from build123d import *

# Parameters (mm, degrees)
SKETCH1_W           = 42
SKETCH1_H           = 47
BOSS_EXTRUDE1_DEPTH = 5
SKETCH2_R           = 1.5
SKETCH2_R_2         = 12.5
CUT_EXTRUDE1_DEPTH  = 32.910029771
SKETCH4_W           = 42
SKETCH4_H           = 45
BOSS_EXTRUDE2_DEPTH = 5
BOSS_EXTRUDE3_DEPTH = 3
BOSS_EXTRUDE4_DEPTH = 3
SKETCH9_R           = 2
CUT_EXTRUDE4_DEPTH  = 69.373971656
CHAMFER3_SIZE       = 3
CUT_EXTRUDE5_REACH  = 73.903
SKETCH10_R          = 1.5


with BuildPart() as part:
    # Sketch1 → Boss-Extrude1 (new body)
    with BuildSketch(Plane(origin=(0, 0, 0), x_dir=(1, 0, 0), z_dir=(0, 1, 0))):
        Rectangle(SKETCH1_W, SKETCH1_H)
    extrude(amount=BOSS_EXTRUDE1_DEPTH)

    # Sketch2 → Cut-Extrude1 (cut, through all)
    with BuildSketch(Plane(origin=(0, 5, 0), x_dir=(1, 0, 0), z_dir=(0, 1, 0))):
        with Locations(Location((-15.5, 13, 0), (0, 0, 270))):
            Circle(SKETCH2_R)
        with Locations(Location((15.5, 13, 0), (0, 0, 270))):
            Circle(SKETCH2_R)
        with Locations(Location((15.5, -18, 0), (0, 0, 270))):
            Circle(SKETCH2_R)
        with Locations(Location((-15.5, -18, 0), (0, 0, 270))):
            Circle(SKETCH2_R)
        with Locations(Location((0, -2.5, 0), (0, 0, 270))):
            Circle(SKETCH2_R_2)
    extrude(amount=-CUT_EXTRUDE1_DEPTH, mode=Mode.SUBTRACT)

    # Sketch4 → Boss-Extrude2 (add)
    with BuildSketch(Plane(origin=(0, 0, -23.5), x_dir=(-1, 0, 0), z_dir=(0, 0, -1))):
        with Locations((0, 22.5)):
            Rectangle(SKETCH4_W, SKETCH4_H)
    extrude(amount=BOSS_EXTRUDE2_DEPTH)

    # Sketch5 → Boss-Extrude3 (add)
    with BuildSketch(Plane(origin=(21, 0, 0), x_dir=(0, 0, -1), z_dir=(1, 0, 0))):
        Polygon((23.5, 13), (15.5, 5), (23.5, 5), align=None)
    extrude(amount=-BOSS_EXTRUDE3_DEPTH)

    # Sketch6 → Boss-Extrude4 (add)
    with BuildSketch(Plane.ZY.offset(21)):
        Polygon((-23.5, 13), (-15.5, 5), (-23.5, 5), align=None)
    extrude(amount=-BOSS_EXTRUDE4_DEPTH)

    # Sketch9 → Cut-Extrude4 (cut, through all)
    with BuildSketch(Plane.XY.offset(-23.5)):
        with Locations((-12.5, 37.5)):
            Circle(SKETCH9_R)
        with Locations((12.5, 37.5)):
            Circle(SKETCH9_R)
        with Locations((12.5, 12.5)):
            Circle(SKETCH9_R)
        with Locations((-12.5, 12.5)):
            Circle(SKETCH9_R)
    extrude(amount=-CUT_EXTRUDE4_DEPTH, mode=Mode.SUBTRACT)

    # Chamfer3
    chamfer3_edges = [part.edges().sort_by_distance(p)[0] for p in [
        (-21, 2.5, 23.5),
        (21, 2.5, 23.5),
        (21, 45, -26),
        (-21, 45, -26),
    ]]
    chamfer(chamfer3_edges, length=CHAMFER3_SIZE)

    # Sketch10 → Cut-Extrude5 (cut, up to next)
    with BuildSketch(Plane(origin=(0, 0, -28.5), x_dir=(-1, 0, 0), z_dir=(0, 0, -1)), mode=Mode.PRIVATE) as cut_extrude5_sk1:
        with Locations((0, 30)):
            Circle(SKETCH10_R)
    cut_extrude5_tool1 = extrude(cut_extrude5_sk1.sketch, amount=-CUT_EXTRUDE5_REACH, mode=Mode.PRIVATE) & part.part
    # Sketch10 → Cut-Extrude5 (cut, up to next)
    with BuildSketch(Plane(origin=(0, 0, -28.5), x_dir=(-1, 0, 0), z_dir=(0, 0, -1)), mode=Mode.PRIVATE) as cut_extrude5_sk2:
        with Locations((0, 15)):
            Circle(SKETCH10_R)
    cut_extrude5_tool2 = extrude(cut_extrude5_sk2.sketch, amount=-CUT_EXTRUDE5_REACH, mode=Mode.PRIVATE) & part.part
    add(cut_extrude5_tool1.solids().sort_by_distance((0, 30, -28.5))[0], mode=Mode.SUBTRACT)
    add(cut_extrude5_tool2.solids().sort_by_distance((0, 15, -28.5))[0], mode=Mode.SUBTRACT)


solid = part.part
Verification items for the finished model (mm, model axes). A direction names the side the tool comes from. Give positions to 0.01 mm unless a question says otherwise; leave off trailing zeros. Write each loop counter-clockwise with the first axis right and the second up, starting at its lowest first coordinate (ties: lowest second). Pieces come first, ordered by that corner, then holes. Notation, with made-up numbers: M 62,14 L 97,14 A30 cw 97,44 Z; hole C 7,33 d4. An arc over 180 degrees is marked long. Put each result on its own line as item: value. Start each with the question number.
1. Go/stop test with flat-tipped pins: pin 1 Ø2 at (x, y) = (8.5, 12) entering from +Z; pin 2 Ø4 at (x, z) = (-15.5, 18) entering from +Y. Record where each tip stops, or that it passes through.
2. Section check A-A (x = 7.5). Record the cut outline in (y, z).
3. Section check B-B (y = 37.5). Record the cut outline in (x, z).
4. Section check D-D (z = 2.5). Record the cut outline in (x, y), and give its area (3 significant figures).
5. Draft check along Y on faces 1 (the face through (-12.934, 35.548, -25.965)), 2 (the face through (3.755, 2.535, 14.423)), 3 (the face through (-19, 44, -26)), 4 (the face through (-9, 0, -8)). Enter one of: +Y half, -Y half, draft (parallel to the pull), parting line (faces both ways), or undercut.
6. Section check C-C (z = 18). Record the cut outline in (x, y), and give its area (3 significant figures).
7. Scan lines: line 1 along X through (y, z) = (3.65, -13); line 2 along Y through (x, z) = (-12.5, -26.5); line 3 along Z through (x, y) = (14.5, 3). Record each from-to range of solid material in increasing order. Write a range as [from, to].
8. Set-up check for faces 5 (the face through (-10, 5, -6)), 6 (the face through (-19.5, 9.1, -19.6)): record each of +Z, -Z, +X, -X, +Y, -Y from which the full face is reachable in a straight line by a thin tool's end or side.
Answer list:
1. pin 1: z = -23.5
1. pin 2: y = 5
2. outline: M 0,-28.5 L 45,-28.5 L 45,-23.5 L 5,-23.5 L 5,-7.5 L 0,-7.5 Z; M 0,12.5 L 5,12.5 L 5,23.5 L 0,23.5 Z
3. outline: M -21,-28.5 L -14.5,-28.5 L -14.5,-23.5 L -21,-23.5 Z; M -10.5,-28.5 L 10.5,-28.5 L 10.5,-23.5 L -10.5,-23.5 Z; M 14.5,-28.5 L 21,-28.5 L 21,-23.5 L 14.5,-23.5 Z
4. outline: M -21,0 L -12.5,0 L -12.5,5 L -21,5 Z; M 12.5,0 L 21,0 L 21,5 L 12.5,5 Z
4. area: 85.0 mm2
5. face 1: undercut
5. face 2: draft
5. face 3: +Y half
5. face 4: -Y half
6. outline: M -21,0 L -17,0 L -17,5 L -21,5 Z; M -14,0 L 14,0 L 14,5 L -14,5 Z; M 17,0 L 21,0 L 21,5 L 17,5 Z
6. area: 180 mm2
7. line 1: [-21, -17], [-14, 14], [17, 21]
7. line 2: [0, 10.5], [14.5, 35.5], [39.5, 45]
7. line 3: [-28.5, -14.12], [-11.88, 16.88], [19.12, 23.5]
8. face 5: +Z, +Y
8. face 6: +Z, +X, -X, +Y
